Autodesk Inventor part; units mm, degrees
ref_plane "YZ Plane" through (0, 0, 0) normal (1, 0, 0) x (0, 1, 0)
ref_plane "XZ Plane" through (0, 0, 0) normal (0, 1, 0) x (-1, 0, 0)
ref_plane "XY Plane" through (0, 0, 0) normal (0, 0, 1) x (1, 0, 0)
sketch "Sketch1" plane through (0, 0, 0) normal (0, 0, 1) x (1, 0, 0)
  circle A0 centre (0, 0) radius 16.5
  dimension "d0" = 33
extrude "Extrusion1" add sketch "Sketch1" along normal blind 22
sketch "Sketch2" plane through (0, 0, 22) normal (0, 0, 1) x (1, 0, 0)
  circle A0 centre (0, 0) radius 16.5
  circle A1 centre (0, 0) radius 18.5
  dimension "d4" = 37
extrude "Extrusion2" add sketch "Sketch2" along normal blind 22 contours A0 | A1
sketch "Sketch3" plane through (0, 0, 44) normal (0, 0, 1) x (1, 0, 0)
  circle A0 centre (0, 7) radius 6
  point P0 (0, 0)
  dimension "d7" = 12
  dimension "d8" = 7
extrude "Extrusion3" add sketch "Sketch3" along normal blind 6
sketch "Sketch4" plane through (0, 7, 50) normal (0, 0, 1) x (1, 0, 0)
  circle A0 centre (0, 0) radius 3
  circle A1 centre (0, 0) radius 6 construction
  point P0 (0, -7)
  dimension "d11" = 6
extrude "Extrusion4" add sketch "Sketch4" along normal blind 3
sketch "Sketch5" plane through (0, 7, 53) normal (0, 0, 1) x (1, 0, 0)
  circle A0 centre (0, 0) radius 3
  circle A1 centre (0, 0) radius 3
  line L0 (-2.0396, -2.2) -> (2.0396, -2.2)
  point P0 (0, -7)
  dimension "d14" = 5.2
extrude "Extrusion5" add sketch "Sketch5" along normal blind 12 contours A0 L0 picked at (0.0839, -0.4702)
chamfer "Chamfer1" distance 0.5 angle 45 2 edges at (0, 10, 65) (0, 4.8, 65)
sketch "Sketch6" plane through (0, 0, 44) normal (0, 0, 1) x (1, 0, 0)
  circle A0 centre (0, 0) radius 15.5 construction
  line L0 (0, -25.9) -> (0, 25.9) construction
  point P0 (15.5, 0)
  point P1 (-15.5, 0)
  point P2 (-7.75, -13.4234)
  point P3 (7.75, 13.4234)
  point P4 (7.75, -13.4234)
  point P5 (-7.75, 13.4234)
  dimension "d20" = 31
  dimension "d23" = 120
hole "Hole1" at (15.5, 0, 44) at (-15.5, 0, 44) at (-7.75, -13.4234, 44) at (7.75, 13.4234, 44) at (7.75, -13.4234, 44) at (-7.75, 13.4234, 44) direction (0, 0, -1) diameter 3.2 depth 3.5 tip angle 118
properties part number "12v DC motor"
Design review of the part built by this model. Coordinates are the model's own, in mm. A direction names the side the tool comes from. Round coordinates to 2 decimals unless told otherwise and drop trailing zeros. Write each loop counter-clockwise with the first axis right and the second up, starting at its lowest first coordinate (ties: lowest second). Pieces come first, ordered by that corner, then holes. Notation, with made-up numbers: (-35.75, 1.5) -> (1.25, 1.5) arc R20 cw to (1.25, 26.5) -> close; hole circle Ø6 at (0.5, 68). An arc over 180 degrees is marked (long way). One line per item, written item: value. Start each with the question number.
Q1. Add section B-B (y = 2.5). Give the boundary of the cut face in (x, z), then the cut area to 3 significant figures.
Q2. Add section A-A (x = 0). Give the boundary of the cut face in (y, z), then the cut area to 3 significant figures.
Q3. Insertion check: P1, Ø6, axis at x = -11, z = 33.5, coming from the +Y side; P2, Ø10, axis at x = -5, z = 51.5, coming from the -Y side; P3, Ø3.5, axis at x = 0, y = 5, coming from the +Z side; P4, Ø5, axis at y = 15, z = 34.5, coming from the -X side. Each pin has a flat end and moves straight along its axis. Give the tip position at first contact, or say it passes through.
Q4. Add section D-D (x = -11.5). Give the boundary of the cut face in (y, z).
Q5. The part is to be moulded in two halves that separate along X. For faces 4 (the face through (-7.562, 13.628, 39.706)), 5 (the face through (0, 4.8, 59)), 6 (the face through (-6, 7, 47)), say which applies: pulls with the +X half, pulls with the -X half, needs draft (parallel to the pull), parting line crosses it, or undercut.
Q6. Add section C-C (z = 54). Give the boundary of the cut face in (x, y), then the cut area to 3 significant figures.
Q7. Tool access review of faces 1 (the face through (9.17, -14.16, 42.23)), 2 (the face through (0, 7, 65)), 3 (the face through (15.24, 6.32, 10.85)): name each direction out of +Z, -Z, +X, -X, +Y, -Y from which nothing blocks a thin tool from reaching the whole face with its end or side.
Q8. To check wall thickness, follow probe 1 along Y at (x, z) = (7, 42); probe 2 along Y at (x, z) = (-7.75, 43); probe 3 along Z at (x, y) = (-6, 9). State the ranges of each line that lie inside material, in increasing order.
Response:
1. outline: (-18.33, 22) -> (-16.31, 22) -> (-16.31, 0) -> (16.31, 0) -> (16.31, 22) -> (18.33, 22) -> (18.33, 44) -> (3.97, 44) -> (3.97, 50) -> (-3.97, 50) -> (-3.97, 44) -> (-18.33, 44) -> close
1. area: 1,570 mm^2
2. outline: (-18.5, 22) -> (-16.5, 22) -> (-16.5, 0) -> (16.5, 0) -> (16.5, 22) -> (18.5, 22) -> (18.5, 44) -> (13, 44) -> (13, 50) -> (10, 50) -> (10, 64.5) -> (9.5, 65) -> (5.3, 65) -> (4.8, 64.5) -> (4.8, 53) -> (4, 53) -> (4, 50) -> (1, 50) -> (1, 44) -> (-18.5, 44) -> close
2. area: 1,690 mm^2
3. P1: stops at y = 16.68
3. P2: stops at y = 1
3. P3: stops at z = 65
3. P4: stops at x = -13.64
4. outline: (-14.49, 22) -> (-11.83, 22) -> (-11.83, 0) -> (11.83, 0) -> (11.83, 22) -> (14.49, 22) -> (14.49, 44) -> (-14.49, 44) -> close
5. face 4: undercut
5. face 5: needs draft
5. face 6: parting line crosses it
6. outline: (-2.04, 4.8) -> (2.04, 4.8) arc R3 ccw (long way) to start
6. area: 26.0 mm^2
7. face 1: +Z
7. face 2: +Z, +X, -X, +Y, -Y
7. face 3: -Z
8. probe 1: y = -17.12 to -14.84, -12.01 to 12.01, 14.84 to 17.12
8. probe 2: y = -16.8 to -15.02, -11.82 to 11.82, 15.02 to 16.8
8. probe 3: z = 0 to 44
